For this review, use the dimensioned drawing (mm, ordinates from the lowest corner) and the shaded views. Round coordinates to 2 decimals unless told otherwise and drop trailing zeros. Write each loop counter-clockwise with the first axis right and the second up, starting at its lowest first coordinate (ties: lowest second). Pieces come first, ordered by that corner, then holes.
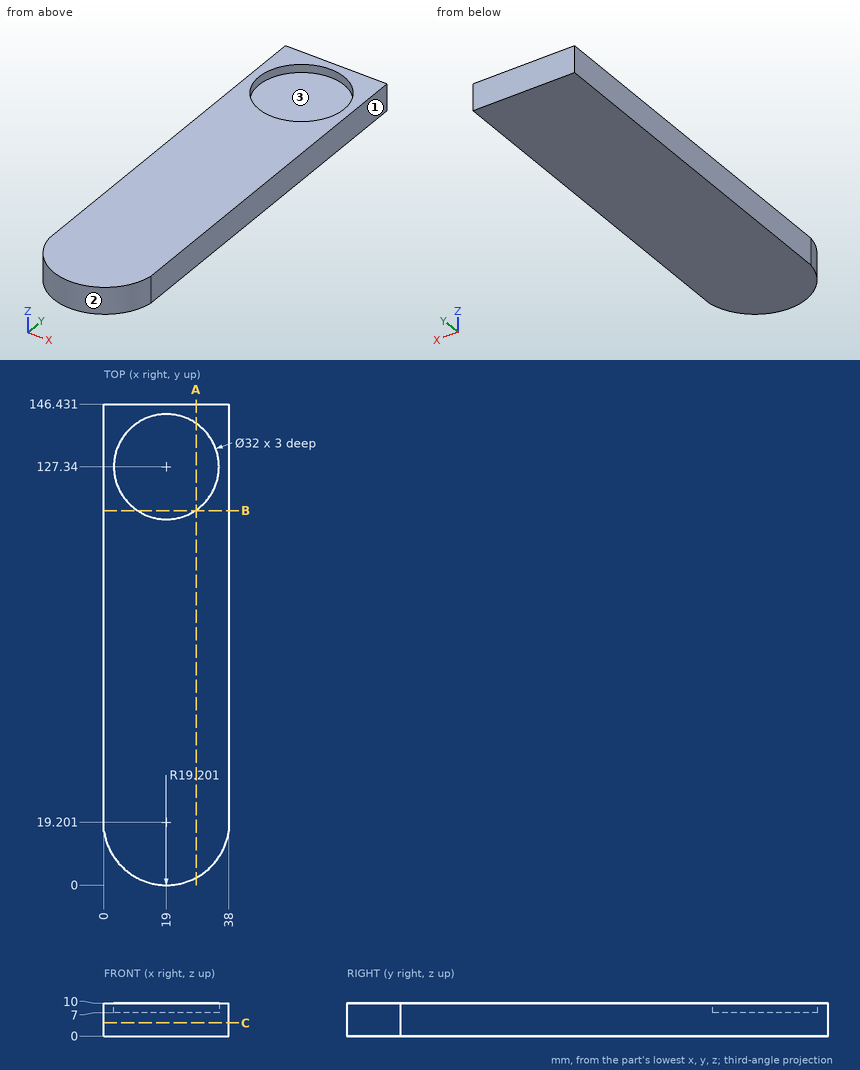
(1) We need section C-C, the plane z = 4. Give the boundary of the cut face in (x, y).
Geometry check:
outline: (0, 16.43) arc R19.2 ccw to (38, 16.43) - (38, 146.43) - (0, 146.43) - close
(2) We need section B-B, the plane y = 114. Give the boundary of the cut face in (x, z).
Geometry check:
outline: (0, 0) - (38, 0) - (38, 10) - (27.83, 10) - (27.83, 7) - (10.17, 7) - (10.17, 10) - (0, 10) - close
(3) For line 1 along Y through (x, z) = (19, 7.9); line 2 along Z through (x, y) = (20.5, 112); line 3 along Y through (x, z) = (19.5, 0.5), list the stretches that pass through material, from the lowest coordinate up.
Geometry check:
line 1: y = 0 to 111.34, 143.34 to 146.43
line 2: z = 0 to 7
line 3: y = 0.01 to 146.43
(4) Mouldability with a two-part tool opening along Y and no side actions: class the marked faces 1, 2 and 3 as pulls with the +Y half, pulls with the -Y half, needs draft (parallel to the pull), parting line crosses it, or undercut.
Geometry check:
face 1: needs draft
face 2: pulls with the -Y half
face 3: undercut
(5) We need section A-A, the plane x = 28. Give the boundary of the cut face in (y, z).
Geometry check:
outline: (2.24, 0) - (146.43, 0) - (146.43, 10) - (140.57, 10) - (140.57, 7) - (114.11, 7) - (114.11, 10) - (2.24, 10) - close
